The listing builds one solid part. Answer for the finished solid, in the listing's coordinates (mm). Face numbers are marked on the shaded views. A direction names the side the tool comes from. Round coordinates to 2 decimals unless told otherwise and drop trailing zeros. Loops run counter-clockwise (first coordinate to the right, second up) from the corner with the lowest first, then second, coordinate; pieces in that order, holes last. Notation, with made-up numbers: (82, 66.25) -> (126, 66.25) arc R28 ccw to (126, 86.25) -> close; hole circle Ø1 at (55.5, -29). An arc over 180 degrees is marked (long way). Answer in a Markdown table with one row per item. Add a question column.
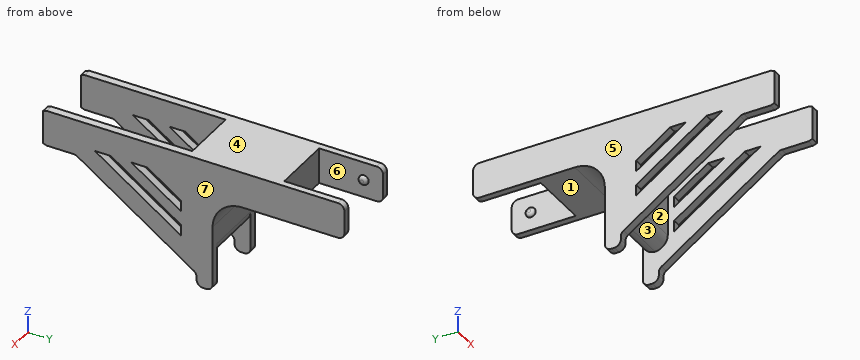
```python
from build123d import *

# Parameters (mm, degrees)
DODANIE_WYCI_GNI_CIE1_DEPTH     = 11.5
SZKIC2_W                        = 9.4
SZKIC2_H                        = 10
SZKIC2_W_2                      = 9
SZKIC2_H_2                      = 24.370303929
WYTNIJ_WYCI_GNI_CIE1_DEPTH      = 36.480417134
WYTNIJ_WYCI_GNI_CIE2_DEPTH      = 36.480417134
WYTNIJ_WYCI_GNI_CIE2_DEPTH_BACK = 36.480417134
SZKIC4_W                        = 9
SZKIC4_H                        = 5
WYTNIJ_WYCI_GNI_CIE3_DEPTH      = 10
ZAOKR_GLENIE1_R                 = 2
ZAOKR_GLENIE2_R                 = 1
SZKIC5_R                        = 0.75
DODANIE_WYCI_GNI_CIE2_DEPTH     = 0.5
ZAOKR_GLENIE3_R                 = 0.5


# Some blends are built 0.0001 mm under size
with BuildPart() as part:
    # Szkic1 → Dodanie-wyciągnięcie1 (new body)
    with BuildSketch(Plane(origin=(0, 0, 0), x_dir=(0, 0, -1), z_dir=(1, 0, 0))):
        with BuildLine():
            Line((0, 0), (-10.3, 0))
            ThreePointArc((-10.3, 0), (-13.623401872, 1.376598128), (-15, 4.7))
            Line((-15, 4.7), (-15, 20.6))
            Line((-15, 20.6), (-20.6, 20.6))
            Line((-20.6, 20.6), (-20.6, -21.4))
            Line((-20.6, -21.4), (-20.6, -25.9))
            Line((-20.6, -25.9), (-20.4, -26.5))
            Line((-20.4, -26.5), (-15.2, -26.5))
            Line((-15.2, -26.5), (-15, -25.9))
            Line((-15, -25.9), (-15, -21.4))
            Line((-15, -21.4), (-2, -2.5))
            Line((-2, -2.5), (0, -2.5))
            Line((0, -2.5), (0, 0))
        make_face()
    extrude(amount=DODANIE_WYCI_GNI_CIE1_DEPTH)

    # Szkic2 → Wytnij-wyciągnięcie1 (cut, through all)
    with BuildSketch(Plane.XY.offset(20.6)):
        with Locations((5.75, 15.6)):
            Rectangle(SZKIC2_W, SZKIC2_H)
        with Locations((5.75, -16.085151964)):
            Rectangle(SZKIC2_W_2, SZKIC2_H_2)
    extrude(amount=-WYTNIJ_WYCI_GNI_CIE1_DEPTH, mode=Mode.SUBTRACT)

    # Szkic3 → Wytnij-wyciągnięcie2 (cut, two sides: drawn at the far end of the back side and taken through both)
    with BuildSketch(Plane(origin=(11.5, 0, 0), x_dir=(0, 0, -1), z_dir=(1, 0, 0)).offset(-WYTNIJ_WYCI_GNI_CIE2_DEPTH_BACK)):
        Polygon((-16.6, -12.705585851), (-16.6, -10.198492794), (-12.955534057, -4.9), (-11.231078515, -4.9), align=None)
        Polygon((-16.6, -15.897210923), (-16.6, -18.40430398), (-7.311325305, -4.9), (-9.035780847, -4.9), align=None)
    extrude(amount=WYTNIJ_WYCI_GNI_CIE2_DEPTH + WYTNIJ_WYCI_GNI_CIE2_DEPTH_BACK, mode=Mode.SUBTRACT)

    # Szkic4 → Wytnij-wyciągnięcie3 (cut)
    with BuildSketch(Plane(origin=(0, 0, 0), x_dir=(1, 0, 0), z_dir=(0, 1, 0))):
        with Locations((5.75, -2.5)):
            Rectangle(SZKIC4_W, SZKIC4_H)
    extrude(amount=-WYTNIJ_WYCI_GNI_CIE3_DEPTH, mode=Mode.SUBTRACT)

    # Zaokrąglenie1
    # the kernel refuses this fillet: 2 mm, written as the material it takes off along each edge
    with BuildSketch(Plane(origin=(1.25, -3.9, 5), x_dir=(0, 0, 1), z_dir=(1, 0, 0))) as zaokr_glenie1_piece_1:
        with BuildLine():
            CenterArc((ZAOKR_GLENIE1_R, -ZAOKR_GLENIE1_R), ZAOKR_GLENIE1_R, 90, 90)
            Line((0, -ZAOKR_GLENIE1_R), (0, 0))
            Line((0, 0), (ZAOKR_GLENIE1_R, 0))
        make_face()
    extrude(amount=9, mode=Mode.SUBTRACT)
    with BuildSketch(Plane(origin=(1.25, 0, 5), x_dir=(0, 0, 1), z_dir=(1, 0, 0))) as zaokr_glenie1_piece_2:
        with BuildLine():
            CenterArc((ZAOKR_GLENIE1_R, ZAOKR_GLENIE1_R), ZAOKR_GLENIE1_R, 180, 90)
            Line((0, ZAOKR_GLENIE1_R), (0, 0))
            Line((0, 0), (ZAOKR_GLENIE1_R, 0))
        make_face()
    extrude(amount=9, mode=Mode.SUBTRACT)

    # Zaokrąglenie2
    zaokr_glenie2_edges = [part.edges().sort_by_distance(p)[0] for p in [
        (0.625, 0, 0),
        (0.625, -2.5, 0),
        (0.625, -2.5, 2),
        (10.975, 20.6, 20.6),
        (10.975, 20.6, 15),
        (10.875, 0, 0),
        (10.875, -2.5, 0),
        (10.875, -2.5, 2),
        (10.875, -21.4, 15),
        (0.525, 20.6, 20.6),
        (0.525, 20.6, 15),
        (0.625, -21.4, 15),
    ]]
    fillet(zaokr_glenie2_edges, radius=ZAOKR_GLENIE2_R)

    # Szkic5 → Dodanie-wyciągnięcie2 (add)
    with BuildSketch(Plane.ZY.offset(-10.45)):
        with Locations(Location((17.8, 17.6, 0), (0, 0, 90))):
            Circle(SZKIC5_R)
    extrude(amount=DODANIE_WYCI_GNI_CIE2_DEPTH)

    # Zaokrąglenie3
    zaokr_glenie3_edges = [part.edges().sort_by_distance(p)[0] for p in [
        (9.95, 16.85, 17.8),
    ]]
    fillet(zaokr_glenie3_edges, radius=ZAOKR_GLENIE3_R - 0.0001)  # a hair under: the kernel refuses the full size

    # Lustro2: part across plane


with BuildPart() as part_1:
    add(part.part)
    add(part.part.mirror(Plane(origin=(5.75, 0, 0), x_dir=(0, 0, 1), z_dir=(1, 0, 0))))


solid = part_1.part
```
Item 1: For the marked faces 1, 2 and 3, determine the directions among +Z, -Z, +X, -X, +Y, -Y from which every point of the face is accessible in a straight line to the end or side of a thin tool.
Item 2: Consider L1, parallel to X at y = -5.5, z = 5.5; L2, parallel to Y at x = 4.75, z = 19; L3, parallel to Y at x = 3, z = 13.5. Determine where each line is inside the solid, lowest interval first. Write a range as from..to.
Item 3: The mould has two halves that part along X. Classify the marked faces 4, 5, 6 and 7: +X half, -X half, draft (parallel to the pull), parting line (faces both ways), or undercut.
Item 4: Section A-A, the plane z = 14 is taken. Write down the section's boundary in (x, y).
Item 5: Section C-C, the plane y = -20.5 is taken. Write down the section's boundary in (x, z), and give its area (3 significant figures).
Item 6: Flat-ended cylindrical pins translate along their axes: P1, Ø3, axis at x = 3.5, y = 7.5, coming from the -Z side; P2, Ø1, axis at x = 11, y = -17, coming from the -Z side; P3, Ø5, axis at x = 1.5, z = 10.5, coming from the -Y side. Find the tip coordinate at first contact, or state that the pin passes through.
Item 7: Section D-D, the plane y = 10 is taken. Write down the section's boundary in (x, z), and give its area (3 significant figures).
Item 8: Section B-B, the plane x = 3.25 is taken. Write down the section's boundary in (y, z), and give its area (3 significant figures).
Here are the results:
| question | item | result |
|---|---|---|
| 1 | face 1 | -Z, +X, -X, +Y |
| 1 | face 2 | +Z, -Z, -Y |
| 1 | face 3 | -Z, -Y |
| 2 | L1 | x = 0..1.25, 10.25..11.5 |
| 2 | L2 | y = -3.9..10.6 |
| 2 | L3 | y = -3.9..1.26 |
| 3 | face 4 | draft |
| 3 | face 5 | -X half |
| 3 | face 6 | undercut |
| 3 | face 7 | +X half |
| 4 | outline | (0, -19.95) -> (1.25, -19.95) -> (1.25, -14.62) -> (0, -14.62) -> close; (0, -12.12) -> (1.25, -12.12) -> (1.25, -8.93) -> (0, -8.93) -> close; (0, -6.42) -> (1.25, -6.42) -> (1.25, -3.9) -> (10.25, -3.9) -> (10.25, -6.42) -> (11.5, -6.42) -> (11.5, 1.8) -> (0, 1.8) -> close; (10.25, -19.95) -> (11.5, -19.95) -> (11.5, -14.62) -> (10.25, -14.62) -> close; (10.25, -12.12) -> (11.5, -12.12) -> (11.5, -8.93) -> (10.25, -8.93) -> close |
| 5 | outline | (0, 14.38) -> (1.25, 14.38) -> (1.25, 20.6) -> (0, 20.6) -> close; (10.25, 14.38) -> (11.5, 14.38) -> (11.5, 20.6) -> (10.25, 20.6) -> close |
| 5 | area | 15.5 mm² |
| 6 | P1 | stops at z = 15 |
| 6 | P2 | stops at z = 11.63 |
| 6 | P3 | stops at y = -18.47 |
| 7 | outline | (0, 15) -> (11.5, 15) -> (11.5, 20.6) -> (0, 20.6) -> close |
| 7 | area | 64.4 mm² |
| 8 | outline | (-3.9, 7) arc R2 ccw to (-1.95, 5) arc R2 ccw to (0, 7) -> (0, 10.3) arc R4.7 cw to (4.7, 15) -> (10.6, 15) -> (10.6, 20.6) -> (-3.9, 20.6) -> close |
| 8 | area | 123 mm² |
